The listing builds one solid part. Answer for the finished solid, in the listing's coordinates (mm). Face numbers are marked on the shaded views. A direction names the side the tool comes from. Round coordinates to 2 decimals unless told otherwise and drop trailing zeros. Order: outer loops, then holes, each group sorted by start corner. A loop starts at its lowest first (then second) coordinate and runs counter-clockwise, first axis right, second up. Notation, with made-up numbers: (-24, 53.5) -> (11, 53.5) arc R6 cw to (11, 64.5) -> close; hole circle Ø1 at (10.5, 20.25). An arc over 180 degrees is marked (long way). Return JSON: item names as keys, results as strings. Group by question number.
(1) The part is cut by section D-D (x = 22). Determine the outline of the cut face in (y, z), plus the area to 3 significant figures.
(2) The part is cut by section B-B (y = 8.5). Determine the outline of the cut face in (x, z).
(3) Which of the six approach directions +Z, -Z, +X, -X, +Y, -Y give full straight-line access (tool end or side, diameter ignored) to the marked faces 1, 2 and 3?
(4) The part is cut by section A-A (y = 25.5). Determine the outline of the cut face in (x, z), plus the area to 3 significant figures.
(5) Consider line 1 (X direction, y = 27, z = -1); line 2 (X direction, y = 7.75, z = 2.5) (3 decimals); line 3 (X direction, y = 6, z = 2.75). Determine where each line is inside the solid, lowest interval first. Write a range as [from, to].
(6) Each of these flat-tipped pins is pushed along its axis until it touches: pin 1 (3 mm diameter, centred on y = 4.5, z = 0, fed in from -X); pin 2 (5 mm diameter, centred on x = 36.5, z = 0.5, fed in from +Y). Where does it stop, or does it pass through?
(7) The part is cut by section C-C (z = 2.75). Determine the outline of the cut face in (x, y).
(8) Determine the mould class of the marked faces 4, 5 and 6 for opening direction X: +X half, -X half, draft (parallel to the pull), parting line (faces both ways), or undercut.
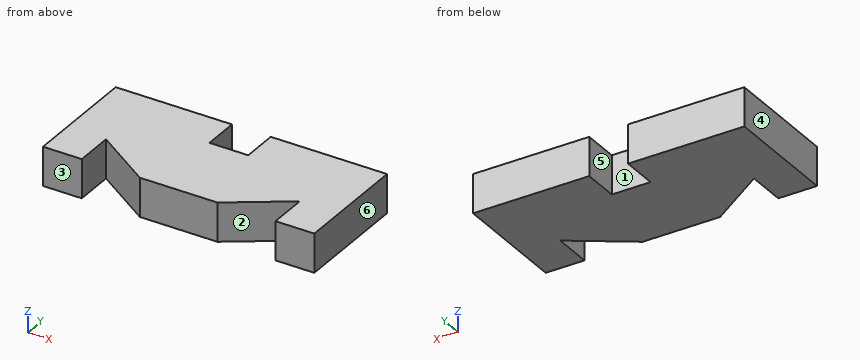
Autodesk Fusion 360 part; units mm, degrees
sketch "Sketch1" plane through (0, 0, 0) normal (0, 0, 1) x (1, 0, 0)
  line L0 (0, 0) -> (0, 30)
  line L1 (0, 30) -> (30, 30)
  line L2 (30, 30) -> (30, 20.7071)
  line L3 (30, 20.7071) -> (40, 20.7071)
  line L4 (40, 20.7071) -> (40, 30)
  line L5 (40, 30) -> (70, 30)
  line L6 (70, 30) -> (70, 0)
  line L7 (60, 0) -> (60, 10)
  line L8 (60, 10) -> (45, 0)
  line L9 (45, 0) -> (25, 0)
  line L10 (25, 0) -> (10, 10)
  line L11 (10, 10) -> (10, 0)
  line L12 (10, 0) -> (0, 0)
  line L13 (60, 0) -> (70, 0)
  dimension "d1" = 30
  dimension "d4" = 30
  dimension "d5" = 30
  dimension "d9" = 70
  dimension "d10" = 10
  dimension "d11" = 15
  dimension "d12" = 20
  dimension "d13" = 10
  dimension "d14" = 15
  dimension "d15" = 10
  dimension "d16" = 30
  dimension "d17" = 10
  dimension "d18" = 10
  dimension "d19" = 20.7071
  dimension "d20" = 90
  dimension "d21" = 112.62
extrude "Extrude1" add sketch "Sketch1" along normal mid plane 10
Answer below:
{
 "1": {"outline": "(2, -5) -> (30, -5) -> (30, 5) -> (2, 5) -> close", "area": "280 mm²"},
 "2": {"outline": "(0, -5) -> (10, -5) -> (10, 5) -> (0, 5) -> close; (12.25, -5) -> (57.75, -5) -> (57.75, 5) -> (12.25, 5) -> close; (60, -5) -> (70, -5) -> (70, 5) -> (60, 5) -> close"},
 "3": {"face 1": "+Z, -Z, +Y", "face 2": "+Z, -Z, -Y", "face 3": "+Z, -Z, +X, -X, -Y"},
 "4": {"outline": "(0, -5) -> (30, -5) -> (30, 5) -> (0, 5) -> close; (40, -5) -> (70, -5) -> (70, 5) -> (40, 5) -> close", "area": "600 mm²"},
 "5": {"line 1": "x = [0, 30], [40, 70]", "line 2": "x = [0, 10], [13.375, 56.625], [60, 70]", "line 3": "x = [0, 10], [16, 54], [60, 70]"},
 "6": {"pin 1": "stops at x = 0", "pin 2": "stops at y = 20.71"},
 "7": {"outline": "(0, 0) -> (10, 0) -> (10, 10) -> (25, 0) -> (45, 0) -> (60, 10) -> (60, 0) -> (70, 0) -> (70, 30) -> (40, 30) -> (40, 20.71) -> (30, 20.71) -> (30, 30) -> (0, 30) -> close"},
 "8": {"face 4": "-X half", "face 5": "undercut", "face 6": "+X half"}
}
